Part model, mm, in its own coordinate system. Face numbers are marked on the shaded views. A direction names the side the tool comes from. Round coordinates to 2 decimals unless told otherwise and drop trailing zeros. Loops run counter-clockwise (first coordinate to the right, second up) from the corner with the lowest first, then second, coordinate; pieces in that order, holes last. Notation, with made-up numbers: M 71,-37.75 L 103,-37.75 A24 ccw 103,-8.75 Z; hole C 52.25,49 d4. An arc over 180 degrees is marked long. Answer as CSV lines item,"result". Start each with the question number.
Item 1: Which spindle directions (+Z, -Z, +X, -X, +Y, -Y) get a long thin tool onto all of the face, cutting with end or side? Do the marked faces 5, 6 and 7. Say none if no direction does.
Item 2: Band-saw the part on C-C (y = 17.5). Give the cut face in (x, z).
Item 3: Band-saw the part on D-D (z = -25). Give the cut face in (x, y).
Item 4: Drop flat-ended pins along their axis: pin 1 Ø4 at (x, y) = (-13.5, 7) entering from -Z; pin 2 Ø5 at (x, y) = (6, 24.5) entering from +Z; pin 3 Ø2.5 at (y, z) = (17.5, -29.86) entering from +X; pin 4 Ø3 at (x, y) = (16, 27) entering from -Z. Give the stop position or say it passes through.
Item 5: Band-saw the part on B-B (z = 11.5). Give the cut face in (x, y), and give its area (3 significant figures).
Item 6: Wall check: line 1 (Y direction, x = 14.5, z = -6.5); line 2 (X direction, y = 11.5, z = -4.5); line 3 (Z direction, x = 17, y = 10.5). Give the ranges that are in metal, low to high.
Item 7: Band-saw the part on A-A (x = 11). Give the cut face in (y, z), and give its area (3 significant figures).
Item 8: Mould opens along X. For the marked faces 1, 2, 3 and 4 say: pulls with the +X half, pulls with the -X half, needs draft (parallel to the pull), parting line crosses it, or undercut.
```python
from build123d import *

# Parameters (mm, degrees)
SKETCH1_W           = 50
SKETCH1_H           = 60
BOSS_EXTRUDE1_DEPTH = 35
SKETCH2_W           = 44
SKETCH2_H           = 29
CUT_EXTRUDE1_DEPTH  = 30
CUT_EXTRUDE2_DEPTH  = 36
SKETCH5_R           = 1.5
CUT_EXTRUDE3_DEPTH  = 48
CUT_EXTRUDE5_DEPTH  = 50.17
FILLET1_R           = 10
FILLET2_START       = -24.274933135
FILLET2_OUTLINE_W   = 50
FILLET2_OUTLINE_H   = 35
FILLET2_DEPTH       = 10
FILLET2_START_2     = -15.881773092
FILLET2_2_DEPTH     = 35.650922027
FILLET2_3_DEPTH     = 25
FILLET2_START_3     = 10
FILLET2_4_DEPTH     = 15
FILLET2_5_ANGLE     = 90


with BuildPart() as part:
    # Sketch1 → Boss-Extrude1 (new body)
    with BuildSketch(Plane(origin=(0, 0, 0), x_dir=(1, 0, 0), z_dir=(0, 1, 0))):
        with Locations((0, 10.230851065)):
            Rectangle(SKETCH1_W, SKETCH1_H)
    extrude(amount=BOSS_EXTRUDE1_DEPTH)

    # Sketch2 → Cut-Extrude1 (cut)
    with BuildSketch(Plane.XY.offset(19.769148935)):
        with Locations((0, 17.5)):
            Rectangle(SKETCH2_W, SKETCH2_H)
    extrude(amount=-CUT_EXTRUDE1_DEPTH, mode=Mode.SUBTRACT)

    # Sketch4 → Cut-Extrude2 (cut)
    with BuildSketch(Plane(origin=(0, 0, 0), x_dir=(-1, 0, 0), z_dir=(0, -1, 0))):
        Polygon((-25, 24.274933135), (-21.25, 24.274933135), (-21.25, 40.230851065), (-6.25, 40.230851065), (-6.25, 24.274933135), (6.25, 24.274933135), (6.25, 40.230851065), (21.25, 40.230851065), (21.25, 24.274933135), (25, 24.274933135), (38.228638219, 24.274933135), (38.228638219, 61.695696762), (-27.361816785, 61.695696762), (-27.361816785, 24.274933135), align=None)
    extrude(amount=-CUT_EXTRUDE2_DEPTH, mode=Mode.SUBTRACT)

    # Sketch5 → Cut-Extrude3 (cut)
    with BuildSketch(Plane(origin=(21.25, 0, 0), x_dir=(0, 0, -1), z_dir=(1, 0, 0))):
        with Locations((29.859024855, 17.5)):
            Circle(SKETCH5_R)
    extrude(amount=-CUT_EXTRUDE3_DEPTH, mode=Mode.SUBTRACT)

    # Sketch12 → Cut-Extrude5 (cut)
    with BuildSketch(Plane.ZY.offset(21.25)):
        Polygon((-40.230851065, 10), (-24.274933135, 10), (-24.274933135, -4.872452702), (-41.905821838, -4.872452702), (-41.905821838, 36.918280203), (-24.274933135, 36.918280203), (-24.274933135, 25), (-40.230851065, 25), align=None)
    extrude(amount=-CUT_EXTRUDE5_DEPTH, mode=Mode.SUBTRACT)

    # Fillet1
    fillet1_edges = [part.edges().sort_by_distance(p)[0] for p in [
        (0, 35, -24.274933135),
    ]]
    fillet(fillet1_edges, radius=FILLET1_R - 0.0001)  # a hair under: the kernel refuses the full size

    # Fillet2: read off the stored shape, not the designer's step
    # Fillet2 outline → Fillet2 (cut)
    with BuildSketch(Plane.XY.offset(FILLET2_START)):
        with Locations((0, 17.5)):
            Rectangle(FILLET2_OUTLINE_W, FILLET2_OUTLINE_H)
    extrude(amount=FILLET2_DEPTH, mode=Mode.SUBTRACT)

    # Fillet2 2 outline → Fillet2 2 (cut)
    with BuildSketch(Plane.XY.offset(FILLET2_START_2)):
        with BuildLine():
            Line((25, 35), (15, 35))
            ThreePointArc((15, 35), (22.071067812, 32.071067812), (25, 25))
            Line((25, 25), (25, 35))
        make_face()
        with BuildLine():
            ThreePointArc((-25, 25), (-22.071067812, 32.071067812), (-15, 35))
            Line((-15, 35), (-25, 35))
            Line((-25, 35), (-25, 25))
        make_face()
    extrude(amount=FILLET2_2_DEPTH, mode=Mode.SUBTRACT)

    # Fillet2 3 outline → Fillet2 3 (add)
    with BuildSketch(Plane(origin=(0, 0, 0), x_dir=(1, 0, 0), z_dir=(0, 1, 0))):
        with BuildLine():
            ThreePointArc((-15, 24.274933135), (-22.071067812, 21.346000947), (-25, 14.274933135))
            Line((-25, 14.274933135), (25, 14.274933135))
            ThreePointArc((25, 14.274933135), (22.071067812, 21.346000947), (15, 24.274933135))
            Line((15, 24.274933135), (-15, 24.274933135))
        make_face()
    extrude(amount=FILLET2_3_DEPTH)

    # Fillet2 4 outline → Fillet2 4 (add)
    with BuildSketch(Plane(origin=(0, 0, 0), x_dir=(1, 0, 0), z_dir=(0, 1, 0)).offset(FILLET2_START_3)):
        with BuildLine():
            Line((-21.25, 24.274933135), (-21.25, 22.081180633))
            ThreePointArc((-21.25, 22.081180633), (-18.311912214, 23.710569706), (-15, 24.274933135))
            Line((-15, 24.274933135), (-21.25, 24.274933135))
        make_face()
        with BuildLine():
            ThreePointArc((15, 24.274933135), (18.311912214, 23.710569706), (21.25, 22.081180633))
            Line((21.25, 22.081180633), (21.25, 24.274933135))
            Line((21.25, 24.274933135), (15, 24.274933135))
        make_face()
    extrude(amount=FILLET2_4_DEPTH)

    # Fillet2 5 outline → Fillet2 5 (revolve)
    with BuildSketch(Plane(origin=(0, 25, -14.274933135), x_dir=(0, 0, -1), z_dir=(0, -1, 0))):
        with BuildLine():
            Line((10, -15), (10, 15))
            ThreePointArc((10, 15), (7.071067812, 22.071067812), (0, 25))
            Line((0, 25), (0, -25))
            ThreePointArc((0, -25), (7.071067812, -22.071067812), (10, -15))
        make_face()
    revolve(axis=Axis((0, 25, -14.274933135), (1, 0, 0)), revolution_arc=FILLET2_5_ANGLE)


solid = part.part
```
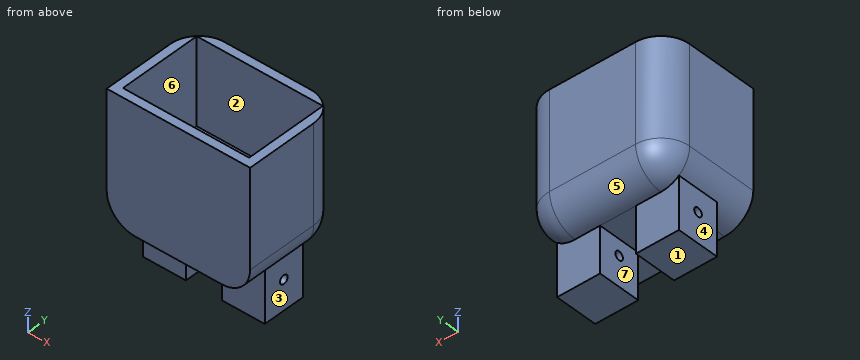
Answer block:
1,face 5,"-Z, +X, -X, +Y"
1,face 6,"+Z"
1,face 7,"-Z, +Y, -Y"
2,outline,"M -25,-14.27 A10 ccw -21.25,-22.08 L -21.25,-28.36 L -6.25,-28.36 L -6.25,-24.27 L 6.25,-24.27 L 6.25,-28.36 L 21.25,-28.36 L 21.25,-22.08 A10 ccw 25,-14.27 L 25,19.77 L 22,19.77 L 22,-10.23 L -22,-10.23 L -22,19.77 L -25,19.77 Z; M -21.25,-40.23 L -6.25,-40.23 L -6.25,-31.36 L -21.25,-31.36 Z; M 6.25,-40.23 L 21.25,-40.23 L 21.25,-31.36 L 6.25,-31.36 Z"
3,outline,"M -21.25,10 L -6.25,10 L -6.25,25 L -21.25,25 Z; M 6.25,10 L 21.25,10 L 21.25,25 L 6.25,25 Z"
4,pin 1,"stops at z = -24.27"
4,pin 2,"stops at z = -10.23"
4,pin 3,"passes through"
4,pin 4,"stops at z = -24.25"
5,outline,"M -25,0 L 25,0 L 25,25 A10 ccw 15,35 L -15,35 A10 ccw -25,25 Z; hole M -22,3 L 22,3 L 22,32 L -22,32 Z"
5,area,"431 mm^2"
6,line 1,"y = 0 to 3, 32 to 35"
6,line 2,"x = -25 to -22, 22 to 25"
6,line 3,"z = -40.23 to -10.23"
7,outline,"M 0,-24.27 L 10,-24.27 L 10,-40.23 L 25,-40.23 L 25,-24.27 A10 ccw 35,-14.27 L 35,19.77 L 32,19.77 L 32,-10.23 L 3,-10.23 L 3,19.77 L 0,19.77 Z; hole C 17.5,-29.86 d3"
7,area,"882 mm^2"
8,face 1,"needs draft"
8,face 2,"undercut"
8,face 3,"pulls with the +X half"
8,face 4,"pulls with the -X half"
